Input: dimensioned drawing with shaded views. Units: mm. Origin: part minimum x, y, z. Give positions to 0.01 mm unless a question says otherwise; leave off trailing zeros. Write each loop counter-clockwise with the first axis right and the second up, starting at its lowest first coordinate (ties: lowest second). Pieces come first, ordered by that corner, then holes. Notation, with made-up numbers: M 57,46 L 116,46 A8 ccw 116,59 Z; hole C 5.25,40.5 d9. An arc over 180 degrees is marked long. Use CSV: the item, a comma, the result in double quotes. Start each with the question number.
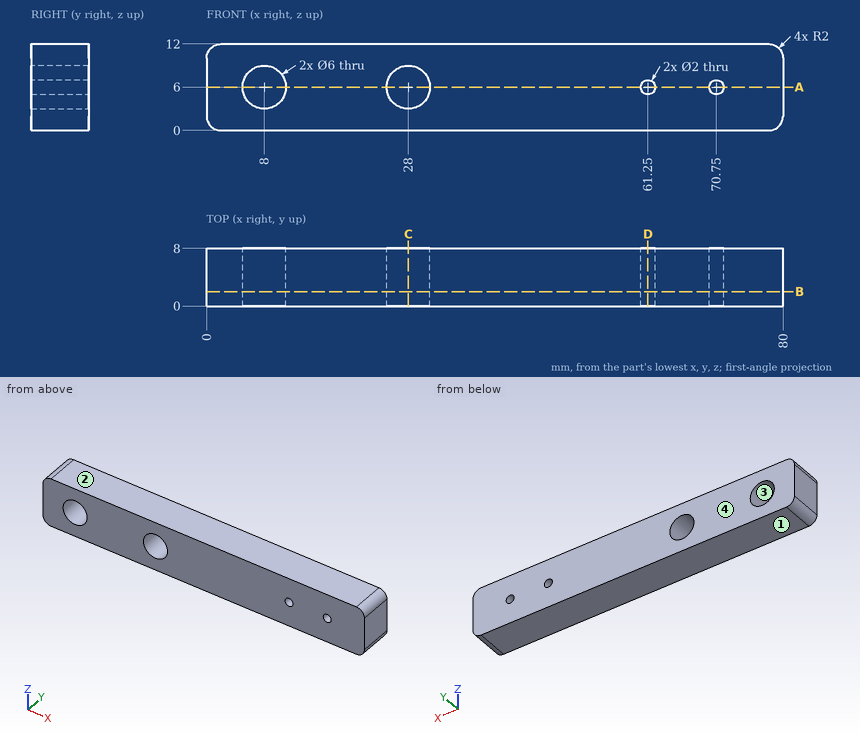
Q1. Section D-D, the plane x = 61.25. Return the cut outline in (y, z), and give its area (3 significant figures).
Q2. Section A-A, the plane z = 6. Return the cut outline in (x, y).
Q3. Pull-direction query (Z, two-part tool) for the marked faces 1, 2, 3 and 4; classes: released by +Z, released by -Z, zero draft, split by the parting line, or undercut.
Q4. Section C-C, the plane x = 28. Return the cut outline in (y, z), and give its area (3 significant figures).
Q5. Section B-B, the plane y = 2. Return the cut outline in (x, z), and give its area (3 significant figures).
Q6. First-contact query: pin 1 Ø2.5 at (x, z) = (70.75, 6) entering from +Y. Flat tip, straight axial feed; report the tip coordinate or a pass-through.
Q7. Material intervals for L1, parallel to X at y = 2.75, z = 6; L2, parallel to Z at x = 70.75, y = 3; L3, parallel to X at y = 6.5, z = 8.5, sorted ascending. Write a range as [from, to].
Check result:
1,outline,"M 0,0 L 8,0 L 8,5 L 0,5 Z; M 0,7 L 8,7 L 8,12 L 0,12 Z"
1,area,"80.0 mm²"
2,outline,"M 0,0 L 5,0 L 5,8 L 0,8 Z; M 11,0 L 25,0 L 25,8 L 11,8 Z; M 31,0 L 60.25,0 L 60.25,8 L 31,8 Z; M 62.25,0 L 69.75,0 L 69.75,8 L 62.25,8 Z; M 71.75,0 L 80,0 L 80,8 L 71.75,8 Z"
3,face 1,"released by -Z"
3,face 2,"released by +Z"
3,face 3,"undercut"
3,face 4,"zero draft"
4,outline,"M 0,0 L 8,0 L 8,3 L 0,3 Z; M 0,9 L 8,9 L 8,12 L 0,12 Z"
4,area,"48.0 mm²"
5,outline,"M 0,2 A2 ccw 2,0 L 78,0 A2 ccw 80,2 L 80,10 A2 ccw 78,12 L 2,12 A2 ccw 0,10 Z; hole C 8,6 d6; hole C 28,6 d6; hole C 61.25,6 d2; hole C 70.75,6 d2"
5,area,"894 mm²"
6,pin 1,"stops at y = 8"
7,L1,"x = [0, 5], [11, 25], [31, 60.25], [62.25, 69.75], [71.75, 80]"
7,L2,"z = [0, 5], [7, 12]"
7,L3,"x = [0, 6.34], [9.66, 26.34], [29.66, 80]"
